Build history of the part. All positions in model axes, mm. A direction names the side the tool comes from. Give positions to 0.01 mm unless a question says otherwise; leave off trailing zeros. Order: outer loops, then holes, each group sorted by start corner. A loop starts at its lowest first (then second) coordinate and runs counter-clockwise, first axis right, second up. Notation, with made-up numbers: M 21.5,79 L 50.5,79 A32 cw 50.5,113 Z; hole C -30.75,16 d11. An arc over 180 degrees is marked long. Answer as CSV lines item,"result".
from build123d import *

# Parameters (mm, degrees)
MODEL_R                 = 1.5
SALIENTE_EXTRUIR1_DEPTH = 3


with BuildPart() as part:
    # Model → Saliente-Extruir1 (new body)
    with BuildSketch(Plane.XY):
        with BuildLine():
            Line((185.972853309, 282.646547335), (178.597853309, 282.646547335))
            Line((178.597853309, 282.646547335), (178.597853309, 264.646547335))
            Line((178.597853309, 264.646547335), (201.097853309, 264.646547335))
            ThreePointArc((201.097853309, 264.646547335), (205.597853309, 269.146547335), (201.097853309, 273.646547335))
            Line((201.097853309, 273.646547335), (189.222853309, 273.646547335))
            ThreePointArc((189.222853309, 273.646547335), (188.07380479, 274.122498816), (187.597853309, 275.271547335))
            Line((187.597853309, 275.271547335), (187.597853309, 281.021547335))
            ThreePointArc((187.597853309, 281.021547335), (187.121901829, 282.170595855), (185.972853309, 282.646547335))
        make_face()
        with Locations((201.097853309, 269.146547335)):
            Circle(MODEL_R, mode=Mode.SUBTRACT)
        with BuildLine():
            Line((182.222853309, 265.896547335), (183.972853309, 265.896547335))
            ThreePointArc((183.972853309, 265.896547335), (184.503183395, 266.116217249), (184.722853309, 266.646547335))
            Line((184.722853309, 266.646547335), (184.722853309, 271.646547335))
            ThreePointArc((184.722853309, 271.646547335), (184.503183395, 272.176877421), (183.972853309, 272.396547335))
            Line((183.972853309, 272.396547335), (182.222853309, 272.396547335))
            ThreePointArc((182.222853309, 272.396547335), (181.692523223, 272.176877421), (181.472853309, 271.646547335))
            Line((181.472853309, 271.646547335), (181.472853309, 266.646547335))
            ThreePointArc((181.472853309, 266.646547335), (181.692523223, 266.116217249), (182.222853309, 265.896547335))
        make_face(mode=Mode.SUBTRACT)
        with BuildLine():
            Line((182.222853309, 274.895968764), (183.972853309, 274.895968764))
            ThreePointArc((183.972853309, 274.895968764), (184.503183395, 275.115638678), (184.722853309, 275.645968764))
            Line((184.722853309, 275.645968764), (184.722853309, 280.645968764))
            ThreePointArc((184.722853309, 280.645968764), (184.503183395, 281.17629885), (183.972853309, 281.395968764))
            Line((183.972853309, 281.395968764), (182.222853309, 281.395968764))
            ThreePointArc((182.222853309, 281.395968764), (181.692523223, 281.17629885), (181.472853309, 280.645968764))
            Line((181.472853309, 280.645968764), (181.472853309, 275.645968764))
            ThreePointArc((181.472853309, 275.645968764), (181.692523223, 275.115638678), (182.222853309, 274.895968764))
        make_face(mode=Mode.SUBTRACT)
    extrude(amount=SALIENTE_EXTRUIR1_DEPTH)


solid = part.part
Item 1: Drop flat-ended pins along their axis: pin 1 (1.5 mm diameter, centred on x = 194.5, z = 1.5, fed in from +Y); pin 2 (1.5 mm diameter, centred on y = 278.5, z = 1, fed in from +X); pin 3 (1.5 mm diameter, centred on y = 272.5, z = 1.5, fed in from +X). Give the stop position or say it passes through.
Geometry says:
pin 1,"stops at y = 273.65"
pin 2,"stops at x = 187.6"
pin 3,"stops at x = 204.77"
Item 2: Band-saw the part on C-C (z = 2). Give the cut face in (x, y) (3 decimals), and give its area (3 significant figures).
Geometry says:
outline,"M 178.598,264.647 L 201.098,264.647 A4.5 ccw 201.098,273.647 L 189.223,273.647 A1.625 cw 187.598,275.272 L 187.598,281.022 A1.625 ccw 185.973,282.647 L 178.598,282.647 Z; hole M 181.473,266.647 A0.75 ccw 182.223,265.897 L 183.973,265.897 A0.75 ccw 184.723,266.647 L 184.723,271.647 A0.75 ccw 183.973,272.397 L 182.223,272.397 A0.75 ccw 181.473,271.647 Z; hole M 181.473,275.646 A0.75 ccw 182.223,274.896 L 183.973,274.896 A0.75 ccw 184.723,275.646 L 184.723,280.646 A0.75 ccw 183.973,281.396 L 182.223,281.396 A0.75 ccw 181.473,280.646 Z; hole C 201.098,269.147 d3"
area,"267 mm2"
Item 3: Band-saw the part on B-B (y = 269.5). Give the cut face in (x, z).
Geometry says:
outline,"M 178.6,0 L 181.47,0 L 181.47,3 L 178.6,3 Z; M 184.72,0 L 199.64,0 L 199.64,3 L 184.72,3 Z; M 202.56,0 L 205.58,0 L 205.58,3 L 202.56,3 Z"
Item 4: 3-axis set-ups, long thin cutter, end or side, ignore diameter. For faces 4 (the flat face through (189, 272, 3)), 5 (the flat face through (183, 265.897, 1)), 6 (the flat face through (195, 273.647, 1)): which of +Z, -Z, +X, -X, +Y, -Y reach the whole face in a straight line?
Geometry says:
face 4,"+Z, +X, -X, +Y, -Y"
face 5,"+Z, -Z"
face 6,"+Z, -Z, +X, +Y"
Item 5: Probe line 1 along X through (y, z) = (269, 1.2); line 2 along X through (y, z) = (277, 0.85); line 3 along X through (y, z) = (270.5, 1.6). List the from-to ranges inside material, lowest first. Write a range as from..to.
Geometry says:
line 1,"x = 178.6..181.47, 184.72..199.61, 202.59..205.6"
line 2,"x = 178.6..181.47, 184.72..187.6"
line 3,"x = 178.6..181.47, 184.72..200.45, 201.74..205.39"
Item 6: Pull direction X, two halves, no side cores. Call faces 1 (the flat face through (183, 281.396, 1)), 2 (the cylindrical face through (188.087, 274.11, 1.479)), 3 (the flat face through (182, 282.647, 1)): released by +X, released by -X, zero draft, split by the parting line, or undercut.
Geometry says:
face 1,"undercut"
face 2,"released by +X"
face 3,"zero draft"
Item 7: Band-saw the part on D-D (x = 196.5). Give the cut face in (y, z).
Geometry says:
outline,"M 264.65,0 L 273.65,0 L 273.65,3 L 264.65,3 Z"
Item 8: Band-saw the part on A-A (y = 277.5). Give the cut face in (x, z).
Geometry says:
outline,"M 178.6,0 L 181.47,0 L 181.47,3 L 178.6,3 Z; M 184.72,0 L 187.6,0 L 187.6,3 L 184.72,3 Z"
